Source: CAD feature listing. Evaluate the final solid. Frame: model axes, mm. A direction names the side the tool comes from. Give positions to 0.01 mm unless a question says otherwise; leave off trailing zeros. Order: outer loops, then holes, each group sorted by start corner. A loop starts at its lowest first (then second) coordinate and runs counter-clockwise, first axis right, second up. Notation, with made-up numbers: (61, -27.5) - (76, -27.5) arc R19 ccw to (76, -0.5) - close; hole circle Ø1 at (-39, -8.75). An arc over 180 degrees is marked (long way). Use CSV: the item, a comma, the result in double quotes.
```python
from build123d import *

# Parameters (mm, degrees)
F1_DEPTH = 4.7625
F2_R     = 1.27


# Not quite as in the source:
# - a length typed as a fraction of an inch, garbled in the dataset ("3 / 203.2 mm" for 3/8 in), is restored


with BuildPart() as f1:
    # F0 (on Top) → F1 (new body)
    with BuildSketch(Plane.XY):
        with BuildLine():
            Line((25.4, 0), (25.4, 5.08))
            Line((25.4, 5.08), (-25.4, 5.08))
            Line((-25.4, 5.08), (-25.4, 0))
            Line((-25.4, 0), (-23.9999255717, 0))
            ThreePointArc((-23.9999255717, 0), (-22.8093005717, 1.190625), (-21.6186755717, 0))
            Line((-21.6186755717, 0), (-19.5611937523, 0))
            ThreePointArc((-19.5611937523, 0), (-18.3705687523, 1.190625), (-17.1799437523, 0))
            Line((-17.1799437523, 0), (18.1277101444, 0))
            ThreePointArc((18.1277101444, 0), (18.3496715251, 1.0652113171), (18.9786101444, 1.9531179662))
            ThreePointArc((18.9786101444, 1.9531179662), (20.7947101444, 2.667), (22.6108101444, 1.9531179662))
            ThreePointArc((22.6108101444, 1.9531179662), (23.2397487637, 1.0652113171), (23.4617101444, 0))
            Line((23.4617101444, 0), (25.4, 0))
        make_face()
        with BuildLine():
            Line((18.1277101444, 0), (18.9786101444, 0))
            Line((18.9786101444, 0), (18.9786101444, 1.9531179662))
            ThreePointArc((18.9786101444, 1.9531179662), (18.3496715251, 1.0652113171), (18.1277101444, 0))
        make_face()
        with BuildLine():
            Line((18.9786101444, -1.9531179662), (18.9786101444, 0))
            Line((18.9786101444, 0), (18.1277101444, 0))
            ThreePointArc((18.1277101444, 0), (18.3496715251, -1.0652113171), (18.9786101444, -1.9531179662))
        make_face()
        with BuildLine():
            Line((22.6108101444, 0), (23.4617101444, 0))
            ThreePointArc((23.4617101444, 0), (23.2397487637, 1.0652113171), (22.6108101444, 1.9531179662))
            Line((22.6108101444, 1.9531179662), (22.6108101444, 0))
        make_face()
        with BuildLine():
            ThreePointArc((22.6108101444, -1.9531179662), (23.2397487637, -1.0652113171), (23.4617101444, 0))
            Line((23.4617101444, 0), (22.6108101444, 0))
            Line((22.6108101444, 0), (22.6108101444, -1.9531179662))
        make_face()
        with BuildLine():
            Line((25.4, -5.08), (25.4, 0))
            Line((25.4, 0), (23.4617101444, 0))
            ThreePointArc((23.4617101444, 0), (23.2397487637, -1.0652113171), (22.6108101444, -1.9531179662))
            ThreePointArc((22.6108101444, -1.9531179662), (20.7947101444, -2.667), (18.9786101444, -1.9531179662))
            ThreePointArc((18.9786101444, -1.9531179662), (18.3496715251, -1.0652113171), (18.1277101444, 0))
            Line((18.1277101444, 0), (-17.1799437523, 0))
            ThreePointArc((-17.1799437523, 0), (-18.3705687523, -1.190625), (-19.5611937523, 0))
            Line((-19.5611937523, 0), (-21.6186755717, 0))
            ThreePointArc((-21.6186755717, 0), (-22.8093005717, -1.190625), (-23.9999255717, 0))
            Line((-23.9999255717, 0), (-25.4, 0))
            Line((-25.4, 0), (-25.4, -5.08))
            Line((-25.4, -5.08), (25.4, -5.08))
        make_face()
    extrude(amount=F1_DEPTH)

    # F2
    f2_edges = [f1.edges().sort_by_distance(p)[0] for p in [
        (25.4, 5.08, 2.38125),
        (25.4, -5.08, 2.38125),
        (-25.4, 5.08, 2.38125),
        (-25.4, -5.08, 2.38125),
    ]]
    fillet(f2_edges, radius=F2_R)


solid = f1.part
```
Item 1: Section A-A on z = 1.95. Return the cut outline in (x, y).
Filled in:
outline,"(-25.4, -3.81) arc R1.27 ccw to (-24.13, -5.08) - (24.13, -5.08) arc R1.27 ccw to (25.4, -3.81) - (25.4, 3.81) arc R1.27 ccw to (24.13, 5.08) - (-24.13, 5.08) arc R1.27 ccw to (-25.4, 3.81) - close; hole circle Ø2.38 at (-22.81, 0); hole circle Ø2.38 at (-18.37, 0); hole (18.98, -1.95) arc R2.67 ccw to (22.61, -1.95) - (22.61, 1.95) arc R2.67 ccw to (18.98, 1.95) - close"
Item 2: Material intervals for line 1 (X direction, y = 0.75, z = 1.45); line 2 (X direction, y = -1, z = 2.25); line 3 (Y direction, x = -18.5, z = 4.35), sorted ascending. Write a range as from..to.
Filled in:
line 1,"x = -25.4..-23.73, -21.88..-19.3, -17.45..18.98, 22.61..25.4"
line 2,"x = -25.4..-23.46, -22.16..-19.02, -17.72..18.98, 22.61..25.4"
line 3,"y = -5.08..-1.18, 1.18..5.08"
Item 3: Mould query, pull axis Y, two halves, no side actions, for faces 1 (the cylindrical face through (20.823, -2.667, 2.348)), 2 (the cylindrical face through (-25.038, -4.698, 2.415)), 3 (the cylindrical face through (25.018, 4.718, 2.415)). Classes: released by +Y, released by -Y, zero draft, split by the parting line, or undercut.
Filled in:
face 1,"undercut"
face 2,"released by -Y"
face 3,"released by +Y"
Item 4: Set-up query: faces 4 (the flat face through (18.979, 0, 2)), 5 (the flat face through (0, -5.08, 2)). Return all of +Z, -Z, +X, -X, +Y, -Y with unobstructed straight access to the full face (end or side cutting, diameter ignored); none if empty.
Filled in:
face 4,"+Z, -Z"
face 5,"+Z, -Z, +X, -X, -Y"
Item 5: First-contact query: pin 1 (1.4 mm diameter, centred on x = -18.37, y = 0, fed in from -Z). Flat tip, straight axial feed; report the tip coordinate or a pass-through.
Filled in:
pin 1,"passes through"
Item 6: Section B-B on y = 0. Return the cut outline in (x, z).
Filled in:
outline,"(-25.4, 0) - (-24, 0) - (-24, 4.76) - (-25.4, 4.76) - close; (-21.62, 0) - (-19.56, 0) - (-19.56, 4.76) - (-21.62, 4.76) - close; (-17.18, 0) - (18.98, 0) - (18.98, 4.76) - (-17.18, 4.76) - close; (22.61, 0) - (25.4, 0) - (25.4, 4.76) - (22.61, 4.76) - close"
